```python
from build123d import *

# Parameters (mm, degrees)
PAD_DEPTH       = 10
POCKET_DEPTH    = 107.501
POCKET001_DEPTH = 53.75
POCKET002_DEPTH = 53.75


with BuildPart() as part:
    # Sketch → Pad (new body)
    with BuildSketch(Plane.XY):
        Polygon((-5, 53.75), (-5, 5), (-53.75, 5), (-53.75, -5), (-5, -5), (-5, -53.75), (5, -53.75), (5, -5), (53.75, -5), (53.75, 5), (5, 5), (5, 53.75), align=None)
    extrude(amount=PAD_DEPTH)

    # Sketch001 → Pocket (cut, through all)
    with BuildSketch(Plane(origin=(0, 53.75, 0), x_dir=(-1, 0, 0), z_dir=(0, 1, 0))):
        with BuildLine():
            ThreePointArc((-2.7, 4.699986), (7e-06, 2), (2.7, 4.7))
            Line((2.7, 10), (2.7, 4.7))
            Line((2.7, 10), (-2.7, 10))
            Line((-2.7, 4.699986), (-2.7, 10))
        make_face()
    extrude(amount=-POCKET_DEPTH, mode=Mode.SUBTRACT)

    # Sketch002 → Pocket001 (cut)
    with BuildSketch(Plane.YZ.offset(53.75)):
        with BuildLine():
            ThreePointArc((-2.7, 4.7), (0, 2), (2.7, 4.700001))
            Line((2.7, 10), (2.7, 4.700001))
            Line((2.7, 10), (-2.7, 10))
            Line((-2.7, 4.7), (-2.7, 10))
        make_face()
    extrude(amount=-POCKET001_DEPTH, mode=Mode.SUBTRACT)

    # Sketch003 → Pocket002 (cut)
    with BuildSketch(Plane(origin=(-53.75, 0, 0), x_dir=(0, -1, 0), z_dir=(-1, 0, 0))):
        with BuildLine():
            ThreePointArc((-2.7, 4.7), (0, 2), (2.7, 4.7))
            Line((2.7, 10), (2.7, 4.7))
            Line((-2.7, 10), (2.7, 10))
            Line((-2.7, 4.7), (-2.7, 10))
        make_face()
    extrude(amount=-POCKET002_DEPTH, mode=Mode.SUBTRACT)


solid = part.part
```
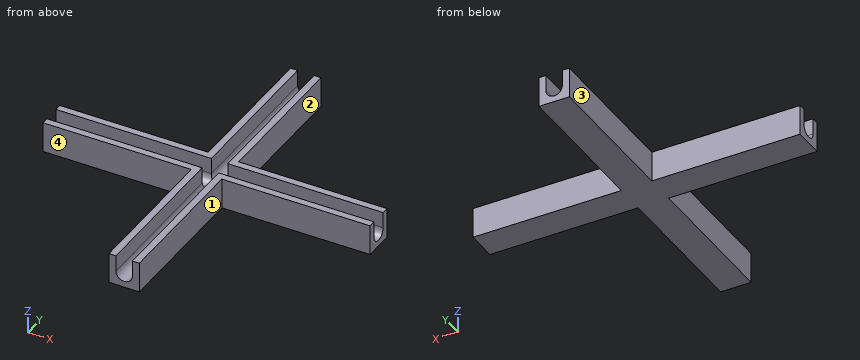
For this review, take the finished solid that the model builds, in its own axes (mm). Face numbers are marked on the shaded views. A direction names the side the tool comes from. Give positions to 0.01 mm unless a question says otherwise; leave off trailing zeros. Order: outer loops, then holes, each group sorted by start corner. A loop starts at its lowest first (then second) coordinate and runs counter-clockwise, first axis right, second up.
1) Take a section at A-A (y = 42). Give the boundary of the cut face in (x, z), then the cut area to 3 significant figures.
2) For the marked faces 1, 2, 3 and 4, list the 3-axis set-ups (+Z, -Z, +X, -X, +Y, -Y) from which the entire face can be reached by the end or side of a thin tool; tool diameter is ignored.
3) Insertion check: pin 1 (2 mm diameter, centred on x = 15, z = 6, fed in from +Y); pin 2 (5 mm diameter, centred on y = 37, z = 6.5, fed in from -X); pin 3 (4 mm diameter, centred on y = -23.5, z = 6.5, fed in from +X). Each pin has a flat end and moves straight along its axis. Give the tip position at first contact, or say it passes through.
4) Wall thickness on line 1 (Y direction, x = -35, z = 6.75); line 2 (X direction, y = 28.5, z = 1): over which ranges is each line inside the solid? List them lowest first.
Derived:
1. outline: (-5, 0) - (5, 0) - (5, 10) - (2.7, 10) - (2.7, 4.7) arc R2.7 cw to (-2.7, 4.7) - (-2.7, 10) - (-5, 10) - close
1. area: 59.9 mm2
2. face 1: +Z, -Z, +X, -Y
2. face 2: +Z, -Z, +X, +Y
2. face 3: +Z, -Z, -X, +Y
2. face 4: +Z, -Z, -X, -Y
3. pin 1: stops at y = 5
3. pin 2: stops at x = -5
3. pin 3: stops at x = 5
4. line 1: y = -5 to -2.7, 2.7 to 5
4. line 2: x = -5 to 5
